Autodesk Inventor part; units mm, degrees
ref_plane "YZ Plane" through (0, 0, 0) normal (1, 0, 0) x (0, 1, 0)
ref_plane "XZ Plane" through (0, 0, 0) normal (0, 1, 0) x (-1, 0, 0)
ref_plane "XY Plane" through (0, 0, 0) normal (0, 0, 1) x (1, 0, 0)
sketch "Sketch1" plane through (0, 0, 0) normal (0, 1, 0) x (-1, 0, 0)
  circle A0 centre (0, 0) radius 38.1
  circle A1 centre (0, 0) radius 5.715
  line L0 (10.4389, 3.81) -> (31.5206, 3.81)
  line L1 (31.5206, -3.81) -> (10.4389, -3.81)
  line L2 (1.9199, 10.9454) -> (12.4607, 29.2026)
  line L3 (19.0598, 25.3926) -> (8.519, 7.1354)
  line L4 (-8.519, 7.1354) -> (-19.0598, 25.3926)
  line L5 (-12.4607, 29.2026) -> (-1.9199, 10.9454)
  line L6 (-10.4389, -3.81) -> (-31.5206, -3.81)
  line L7 (-31.5206, 3.81) -> (-10.4389, 3.81)
  line L8 (-1.9199, -10.9454) -> (-12.4607, -29.2026)
  line L9 (-19.0598, -25.3926) -> (-8.519, -7.1354)
  line L10 (8.519, -7.1354) -> (19.0598, -25.3926)
  line L11 (12.4607, -29.2026) -> (1.9199, -10.9454)
  arc A2 (10.4389, 3.81) -> (8.519, 7.1354) centre (0, 0) ccw
  arc A3 (1.9199, 10.9454) -> (-1.9199, 10.9454) centre (0, 0) ccw
  arc A4 (-8.519, 7.1354) -> (-10.4389, 3.81) centre (0, 0) ccw
  arc A5 (-10.4389, -3.81) -> (-8.519, -7.1354) centre (0, 0) ccw
  arc A6 (-1.9199, -10.9454) -> (1.9199, -10.9454) centre (0, 0) ccw
  arc A7 (8.519, -7.1354) -> (10.4389, -3.81) centre (0, 0) ccw
  arc A8 (19.0598, -25.3926) -> (31.5206, -3.81) centre (0, 0) ccw
  arc A9 (31.5206, 3.81) -> (19.0598, 25.3926) centre (0, 0) ccw
  arc A10 (12.4607, 29.2026) -> (-12.4607, 29.2026) centre (0, 0) ccw
  arc A11 (-19.0598, 25.3926) -> (-31.5206, 3.81) centre (0, 0) ccw
  arc A12 (-31.5206, -3.81) -> (-19.0598, -25.3926) centre (0, 0) ccw
  arc A13 (-12.4607, -29.2026) -> (12.4607, -29.2026) centre (0, 0) ccw
  dimension "d0" = 76.2
  dimension "d1" = 11.43
  dimension "d4" = 3.81
  dimension "d5" = 3.81
  dimension "d8" = 360
  dimension "d10" = 31.75
  dimension "d11" = 11.1125
extrude "Extrusion1" add sketch "Sketch1" along normal blind 12.7
fillet "Fillet1" radius 3.175 24 edges at (-19.0598, 6.35, 25.3926) (-12.4607, 6.35, 29.2026) (12.4607, 6.35, 29.2026) (19.0598, 6.35, 25.3926) (31.5206, 6.35, 3.81) (31.5206, 6.35, -3.81) (19.0598, 6.35, -25.3926) (12.4607, 6.35, -29.2026) (-12.4607, 6.35, -29.2026) (-19.0598, 6.35, -25.3926) (-31.5206, 6.35, -3.81) (-31.5206, 6.35, 3.81) (-8.519, 6.35, 7.1354) (-8.519, 6.35, -7.1354) (-10.4389, 6.35, -3.81) (-10.4389, 6.35, 3.81) (-1.9199, 6.35, 10.9454) (1.9199, 6.35, 10.9454) (8.519, 6.35, 7.1354) (10.4389, 6.35, 3.81) (10.4389, 6.35, -3.81) (8.519, 6.35, -7.1354) (1.9199, 6.35, -10.9454) (-1.9199, 6.35, -10.9454)
properties part number "3in flex"
The model under review builds one solid part; all positions refer to its coordinate system, in mm. A direction names the side the tool comes from. Give positions to 0.01 mm unless a question says otherwise; leave off trailing zeros. Order: outer loops, then holes, each group sorted by start corner. A loop starts at its lowest first (then second) coordinate and runs counter-clockwise, first axis right, second up. Notation, with made-up numbers: M 43,-6.5 L 60,-6.5 A32 cw 60,30.5 Z; hole C -6.75,4 d11. An arc over 180 degrees is marked long. Answer in a Markdown table with one row per item. Add a question column.
1. Machinability: for faces 1 (the flat face through (-8, 0, 1)), 2 (the cylindrical face through (-0.12, 6.26, -31.75)), which of the approach directions +Z, -Z, +X, -X, +Y, -Y give a long, thin tool a straight path to every point of the face, cutting with its end or side? Answer none if there is none.
2. Add section B-B on z = 28.5. State the section outline as (x, y) points.
3. To check wall thickness, follow line 1 along Z through (x, y) = (0, 8) (1 decimal); line 2 along X through (y, z) = (9.75, 0.5); line 3 along Z through (x, y) = (14.5, 9). State the ranges of each line that lie inside material, in increasing order.
4. For pin 1 Ø3 at (y, z) = (8.5, -30) entering from +X; pin 2 Ø6.5 at (x, y) = (18, 7) entering from +Z; pin 3 Ø3 at (x, z) = (-21.5, 21) entering from -Y; pin 4 Ø6.5 at (x, y) = (24, 3.5) entering from -Z, all flat-tipped, find the tip position at first contact; note any pin that passes through.
5. Mouldability with a two-part tool opening along Z and no side actions: class faces 3 (the cylindrical face through (1.732, 6.439, -11.515)), 4 (the flat face through (-8, 12.7, 1)), 5 (the cylindrical face through (30.235, 6.261, 23.183)) as released by +Z, released by -Z, zero draft, split by the parting line, or undercut.
6. Add section A-A on z = 0. State the section outline as (x, y) points (3 decimals), plus the area to 3 significant figures.
7. Add section C-C on y = 4.5. Count the separate pieces of the cut face and the enclosed holes in it, plus the area to 3 significant figures.
The answers:
| question | item | result |
|---|---|---|
| 1 | face 1 | +Z, -Z, +X, -X, -Y |
| 1 | face 2 | +Y, -Y |
| 2 | outline | M -25.29,0 L -10.81,0 L -10.81,12.7 L -25.29,12.7 Z; M 10.81,0 L 25.29,0 L 25.29,12.7 L 10.81,12.7 Z |
| 3 | line 1 | -38.1 to -31.7, -11.1 to -5.7, 5.7 to 11.1, 31.7 to 38.1 |
| 3 | line 2 | -38.1 to -5.69, 5.69 to 38.1 |
| 3 | line 3 | -35.23 to -17.49, -3.81 to 3.81, 17.49 to 35.23 |
| 4 | pin 1 | x = 25.29 |
| 4 | pin 2 | z = 35.13 |
| 4 | pin 3 | through |
| 4 | pin 4 | z = -31.95 |
| 5 | face 3 | undercut |
| 5 | face 4 | zero draft |
| 5 | face 5 | split by the parting line |
| 6 | outline | M -38.1,0 L -5.715,0 L -5.715,12.7 L -38.1,12.7 Z; M 5.715,0 L 38.1,0 L 38.1,12.7 L 5.715,12.7 Z |
| 6 | area | 823 mm2 |
| 7 | separate pieces | 1 |
| 7 | enclosed holes | 7 |
| 7 | area | 2,680 mm2 |
